Autodesk Inventor part; units mm, degrees
ref_plane "YZ Plane" through (0, 0, 0) normal (1, 0, 0) x (0, 1, 0)
ref_plane "XZ Plane" through (0, 0, 0) normal (0, 1, 0) x (-1, 0, 0)
ref_plane "XY Plane" through (0, 0, 0) normal (0, 0, 1) x (1, 0, 0)
sketch "Sketch1" plane through (0, 0, 0) normal (0, 0, 1) x (1, 0, 0)
  line L0 (0, 0) -> (25, 0)
  line L1 (25, 0) -> (25, 10)
  line L2 (25, 10) -> (0, 10)
  line L3 (0, 10) -> (0, 0)
  line L4 (2, 0) -> (10, 0)
  line L5 (10, 0) -> (10, -3)
  line L6 (10, -3) -> (2, -3)
  line L7 (2, -3) -> (2, 0)
  line L8 (12.5, 0) -> (12.5, 10) construction
  line L9 (0, 5) -> (25, 5) construction
  line L10 (15, 0) -> (15, -3)
  line L11 (15, -3) -> (23, -3)
  line L12 (23, -3) -> (23, 0)
  line L13 (10, 10) -> (10, 13)
  line L14 (10, 13) -> (2, 13)
  line L15 (2, 13) -> (2, 10)
  line L16 (15, 13) -> (23, 13)
  line L17 (15, 10) -> (15, 13)
  line L18 (23, 13) -> (23, 10)
  point P0 (23, 0)
  point P1 (15, 0)
  point P2 (10, 0)
  point P3 (15, 10)
  point P4 (23, 10)
  dimension "d0" = 25
  dimension "d1" = 10
  dimension "d5" = 3
  dimension "d6" = 2
  dimension "d7" = 8
extrude "Extrusion1" add sketch "Sketch1" along normal blind 3
properties part number "protector hal"
The listing builds one solid part. Answer for the finished solid, in the listing's coordinates (mm). A direction names the side the tool comes from. Coordinates: 2 decimals unless noted, no trailing zeros. Order: outer loops, then holes, each group sorted by start corner. A loop starts at its lowest first (then second) coordinate and runs counter-clockwise, first axis right, second up. Notation, with made-up numbers: (80.5, 25) -> (92.5, 25) arc R14 cw to (92.5, 43) -> close; hole circle Ø11 at (-0.75, 5.5). An arc over 180 degrees is marked (long way). Answer in a Markdown table with one row per item. Add a question column.
Item 1: Find the intervals of material crossed by L1, parallel to X at y = 10.25, z = 0.7; L2, parallel to Y at x = 14.5, z = 1.05, in increasing order. Write a range as from..to.
Item 2: Which of the six approach directions +Z, -Z, +X, -X, +Y, -Y give full straight-line access (tool end or side, diameter ignored) to faces 4 (the face through (1, 10, 1)), 5 (the face through (1, 0, 1)), 6 (the face through (10, 11, 1))?
Item 3: Each of these flat-tipped pins is pushed along its axis until it touches: P1, Ø1.5, axis at y = 11.5, z = 1.5, coming from the -X side; P2, Ø0.6, axis at x = 0.5, z = 1, coming from the -Y side; P3, Ø0.6, axis at x = 1.5, z = 2, coming from the +Y side. Where does it stop, or does it pass through?
Item 4: Determine the mould class of faces 1 (the face through (15, -1, 1)), 2 (the face through (23, -2, 1)), 3 (the face through (12, 5, 0)) for opening direction X: +X half, -X half, draft (parallel to the pull), parting line (faces both ways), or undercut.
Item 5: Find section A-A (y = -1). Write down the section's boundary in (x, z).
Item 6: Find section B-B (z = 0.7). Write down the section's boundary in (x, y), then the cut area to 3 significant figures.
Result set:
| question | item | result |
|---|---|---|
| 1 | L1 | x = 2..10, 15..23 |
| 1 | L2 | y = 0..10 |
| 2 | face 4 | +Z, -Z, -X, +Y |
| 2 | face 5 | +Z, -Z, -X, -Y |
| 2 | face 6 | +Z, -Z, +Y |
| 3 | P1 | stops at x = 2 |
| 3 | P2 | stops at y = 0 |
| 3 | P3 | stops at y = 10 |
| 4 | face 1 | undercut |
| 4 | face 2 | +X half |
| 4 | face 3 | draft |
| 5 | outline | (2, 0) -> (10, 0) -> (10, 3) -> (2, 3) -> close; (15, 0) -> (23, 0) -> (23, 3) -> (15, 3) -> close |
| 6 | outline | (0, 0) -> (2, 0) -> (2, -3) -> (10, -3) -> (10, 0) -> (15, 0) -> (15, -3) -> (23, -3) -> (23, 0) -> (25, 0) -> (25, 10) -> (23, 10) -> (23, 13) -> (15, 13) -> (15, 10) -> (10, 10) -> (10, 13) -> (2, 13) -> (2, 10) -> (0, 10) -> close |
| 6 | area | 346 mm² |
